Work out the finished part from the listing and answer in its coordinate system (mm). Give positions to 0.01 mm unless a question says otherwise; leave off trailing zeros. Order: outer loops, then holes, each group sorted by start corner. A loop starts at its lowest first (then second) coordinate and runs counter-clockwise, first axis right, second up. Notation, with made-up numbers: (13, -7) - (67, -7) arc R24 cw to (67, 22) - close; hole circle Ø6 at (74, 45). An arc over 180 degrees is marked (long way). Put each result on its own line as item: value.
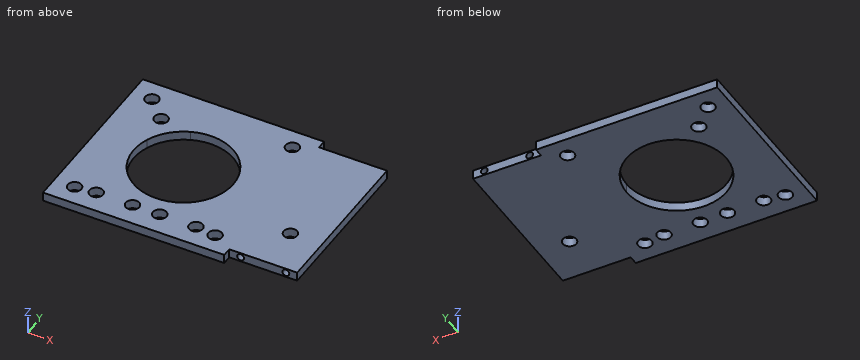
```python
from build123d import *

# Parameters (mm, degrees)
F0_W     = 40
F0_H     = 40
F1_DEPTH = 2
F2_W     = 36
F2_H     = 2
F3_DEPTH = 15
F5_D     = 3
F5_DEPTH = 18
F4_R     = 7
F6_DEPTH = 25
F8_D     = 1.5
F8_DEPTH = 50


with BuildPart() as f1:
    # F0 (on Top) → F1 (new body)
    with BuildSketch(Plane.XY):
        Rectangle(F0_W, F0_H)
    extrude(amount=F1_DEPTH)

    # F2 (on face) → F3 (join)
    with BuildSketch(Plane.YZ.offset(20)):
        with Locations((0, 1)):
            Rectangle(F2_W, F2_H)
    extrude(amount=F3_DEPTH)

    # F5
    with Locations(Plane.XY.offset(2)):
        with Locations((-11, -15), (11, -15), (28, -8), (-11, 11), (-3, -15), (3, -15), (15.5, 15.5), (-15.5, 15.5), (-15.5, -15.5), (15.5, -15.5)):
            Hole(F5_D / 2, depth=F5_DEPTH)

    # F4 (on face) → F6 (cut)
    with BuildSketch(Plane.XY.offset(2)):
        with BuildLine():
            ThreePointArc((-4.042448, 10.230279), (-6.050253, 6.050253), (-10.230279, 4.042448))
            ThreePointArc((-10.230279, 4.042448), (-2.057538, -10.805857), (11, 0))
            ThreePointArc((11, 0), (6.185995, 9.095794), (-4.042448, 10.230279))
        make_face()
        Circle(F4_R, mode=Mode.SUBTRACT)
        Circle(F4_R)
        with BuildLine():
            ThreePointArc((-4.042448, 10.230279), (-7.778175, 7.778175), (-10.230279, 4.042448))
            ThreePointArc((-10.230279, 4.042448), (-6.050253, 6.050253), (-4.042448, 10.230279))
        make_face()
    extrude(amount=-F6_DEPTH, mode=Mode.SUBTRACT)

    # F8
    with Locations(Plane.XZ.offset(18)):
        with Locations((22.5, 1), (32.5, 1)):
            Hole(F8_D / 2, depth=F8_DEPTH)


solid = f1.part
```
(1) Section D-D, the plane y = -8 is taken. Write down the section's boundary in (x, z), then the cut area to 3 significant figures.
Geometry check:
outline: (-20, 0) - (-7.55, 0) - (-7.55, 2) - (-20, 2) - close; (7.55, 0) - (26.5, 0) - (26.5, 2) - (7.55, 2) - close; (29.5, 0) - (35, 0) - (35, 2) - (29.5, 2) - close; hole circle Ø1.5 at (22.5, 1); hole circle Ø1.5 at (32.5, 1)
area: 70.3 mm²
(2) Section C-C, the plane z = 1.4 is taken. Count the separate pieces of the cut face and the enclosed holes in it, then the cut area to 3 significant figures.
Geometry check:
separate pieces: 3
enclosed holes: 11
area: 1,600 mm²
(3) Given pin 1 (4 mm diameter, centred on x = 15.5, y = 15.5, fed in from -Z); pin 2 (1 mm diameter, centred on x = 29.5, z = 1.5, fed in from +Y), each flat-ended and moving along its own axis, determine where each tip first touches the part or whether it passes through.
Geometry check:
pin 1: stops at z = 0
pin 2: stops at y = 18
(4) Section B-B, the plane y = 2.5 is taken. Write down the section's boundary in (x, z), then the cut area to 3 significant figures.
Geometry check:
outline: (-20, 0) - (-10.71, 0) - (-10.71, 2) - (-20, 2) - close; (10.71, 0) - (35, 0) - (35, 2) - (10.71, 2) - close; hole circle Ø1.5 at (22.5, 1); hole circle Ø1.5 at (32.5, 1)
area: 63.6 mm²
(5) Straight lines are drawn through the part: line 1 (Y direction, x = 15.5, z = 1.3); line 2 (Z direction, x = 32.5, y = 10.5); line 3 (Y direction, x = 16.5, z = 1.75). For each, find the intervals that lie inside material, in ascending order.
Geometry check:
line 1: y = -20 to -17, -14 to 14, 17 to 20
line 2: z = 0 to 0.25, 1.75 to 2
line 3: y = -20 to -16.62, -14.38 to 14.38, 16.62 to 20
(6) Section A-A, the plane x = 22.5 is taken. Write down the section's boundary in (y, z).
Geometry check:
outline: (-18, 0) - (18, 0) - (18, 0.25) - (-18, 0.25) - close; (-18, 1.75) - (18, 1.75) - (18, 2) - (-18, 2) - close
